CAD build for the part. Positions are in the model's coordinates, mm. A direction names the side the tool comes from. Coordinates: 2 decimals unless noted, no trailing zeros. Write each loop counter-clockwise with the first axis right and the second up, starting at its lowest first coordinate (ties: lowest second). Pieces come first, ordered by that corner, then holes. Notation, with made-up numbers: (80, 32.25) - (130, 32.25) arc R15 ccw to (130, 60.25) - close; hole circle Ø10 at (-32, 53). An arc over 180 degrees is marked (long way). Answer in a Markdown table with one row per item. Add a question column.
Q1. Band-saw the part on B-B (z = -1.75). List the corners of the cut face in (x, y).
Q2. Two-plate mould, pull along Y, no slides. Class faces 3 (the flat face through (0, 0, 6)), 4 (the conical face through (-17.615, -13.507, -7.691)), 5 (the conical face through (-19, -14, -19)), 6 (the flat face through (0, 0, 3.5)): +Y half, -Y half, draft (parallel to the pull), parting line (faces both ways), or undercut.
Q3. 3-axis set-ups, long thin cutter, end or side, ignore diameter. For faces 1 (the conical face through (-5.356, -24.117, -7.452)), 2 (the cylindrical face through (-6.03, -27.14, 3.99)): which of +Z, -Z, +X, -X, +Y, -Y reach the whole face in a straight line?
Q4. Band-saw the part on C-C (z = -12.25). List the corners of the cut face in (x, y).
Q5. Drill centre lines: line 1 along Z through (x, y) = (16, -19.5); line 2 along Y through (x, z) = (0, -6.25); line 3 along Y through (x, z) = (-15, 4.25). Where is each one in solid material? Low to high. Write a range as from..to.
Q6. Band-saw the part on A-A (x = 0). List the corners of the cut face in (y, z), and give its area (3 significant figures).
Q7. Pin check, flat tips, straight feed: pin 1 (2 mm diameter, centred on x = -11.5, z = -14.5, fed in from -Y); pin 2 (3 mm diameter, centred on y = -16.5, z = -4, fed in from -X); pin 3 (1 mm diameter, centred on y = 20, z = -15.5, fed in from +X); pin 4 (6 mm diameter, centred on x = -9.5, y = 16.5, fed in from -Z). Stop position of each tip, or through.
```python
from build123d import *

# Parameters (mm, degrees)
F0_R          = 24.9
F1_DEPTH      = 19.2
F1_TAPER      = 1.5
F1_DEPTH_BACK = 3
F1_TAPER_BACK = -1.5
F2_R          = 27.8
F3_DEPTH      = 3
F4_SIZE       = 1
F5_T          = -2.5
F6_SIZE       = 1


with BuildPart() as f1:
    # F0 (on Top) → F1 (new body, two sides)
    with BuildSketch(Plane.XY) as f1_sk:
        Circle(F0_R)
    extrude(amount=-F1_DEPTH, taper=F1_TAPER)
    extrude(f1_sk.sketch, amount=F1_DEPTH_BACK, taper=F1_TAPER_BACK)

    # F2 (on face) → F3 (join)
    with BuildSketch(Plane.XY.offset(3)):
        Circle(F2_R)
    extrude(amount=F3_DEPTH)

    # F4
    f4_edges = [f1.edges().sort_by_distance(p)[0] for p in [
        (-27.8, 0, 6),
    ]]
    chamfer(f4_edges, length=F4_SIZE)

    # F5
    f5_openings = [f1.faces().sort_by_distance(p)[0] for p in [
        (0, 0, -19.2),
    ]]
    offset(amount=F5_T, openings=f5_openings, kind=Kind.INTERSECTION)

    # F6
    f6_edges = [f1.edges().sort_by_distance(p)[0] for p in [
        (-24.39723, 0, -19.2),
    ]]
    chamfer(f6_edges, length=F6_SIZE)


solid = f1.part
```
Checked values:
| question | item | result |
|---|---|---|
| 1 | outline | circle Ø49.71 at (0, 0); hole circle Ø44.71 at (0, 0) |
| 2 | face 3 | draft |
| 2 | face 4 | undercut |
| 2 | face 5 | parting line |
| 2 | face 6 | undercut |
| 3 | face 1 | -Z |
| 3 | face 2 | +Z, -Z |
| 4 | outline | circle Ø49.16 at (0, 0); hole circle Ø44.16 at (0, 0) |
| 5 | line 1 | z = 3..6 |
| 5 | line 2 | y = -24.74..-22.24, 22.24..24.74 |
| 5 | line 3 | y = -23.41..23.41 |
| 6 | outline | (-27.8, 3) - (-24.98, 3) - (-24.42, -18.2) - (-23.4, -19.2) - (-21.9, -19.2) - (-22.49, 3.5) - (22.49, 3.5) - (21.9, -19.2) - (23.4, -19.2) - (24.42, -18.2) - (24.98, 3) - (27.8, 3) - (27.8, 5) - (26.8, 6) - (-26.8, 6) - (-27.8, 5) - close |
| 6 | area | 253 mm² |
| 7 | pin 1 | stops at y = -22.16 |
| 7 | pin 2 | stops at x = -19.74 |
| 7 | pin 3 | stops at x = 14.82 |
| 7 | pin 4 | stops at z = -19.2 |
